Here's how the part is built. I have some questions about the finished solid (model axes, mm). Face numbers are marked on the shaded views. Give positions to 0.01 mm unless a question says otherwise; leave off trailing zeros. Write each loop counter-clockwise with the first axis right and the second up, starting at its lowest first coordinate (ties: lowest second). Pieces come first, ordered by that corner, then holes. Notation, with made-up numbers: (64, -32.75) - (81, -32.75) arc R11 cw to (81, -22.75) - close; hole circle Ø9 at (-9.75, -2). An arc over 180 degrees is marked (long way). Write each question's results on one line, items separated by ' | '. Start each with the question number.
Item 1: Suppose I cut it at B-B on z = -70. List the corners of the cut face in (x, y) for me.
Item 2: Will these pins go through, and if not, where does the flat tip stop? P1, Ø5, axis at x = -70, z = -70, coming from the -Y side; P2, Ø1.9, axis at x = -11, z = -11, coming from the +Y side; P3, Ø3, axis at y = 9, z = -67.5, coming from the -X side.
Item 3: Please list where these lines run through material, in increasing order: line 1 along X through (y, z) = (8.75, -70); line 2 along X through (y, z) = (9, -8).
Item 4: Suppose I cut it at A-A on y = 6.5. List the corners of the cut face in (x, z) for me, then the cut area to 3 significant figures.
Item 5: Suppose I cut it at C-C on x = -70. List the corners of the cut face in (y, z) for me, then the cut area to 3 significant figures.
Item 6: We'd pull the mould along X, two halves only. Please class the marked faces 1 and 2: +X half, -X half, draft (parallel to the pull), parting line (faces both ways), or undercut.
Item 7: Suppose I cut it at D-D on z = -16. List the corners of the cut face in (x, y) for me, then the cut area to 3 significant figures.
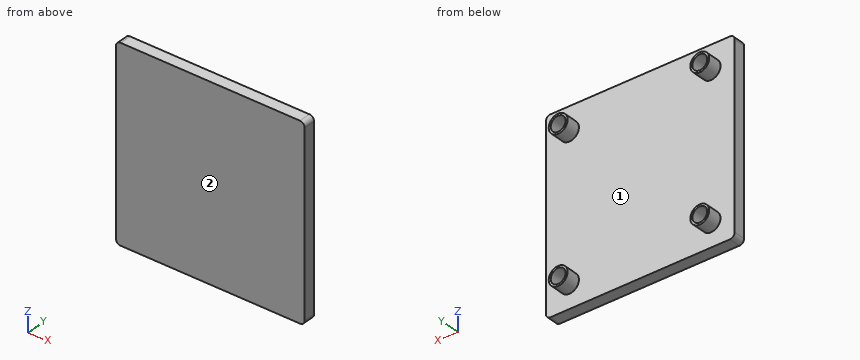
Autodesk Inventor part; units mm, degrees
ref_plane "YZ Plane" through (0, 0, 0) normal (1, 0, 0) x (0, 1, 0)
ref_plane "XZ Plane" through (0, 0, 0) normal (0, 1, 0) x (-1, 0, 0)
ref_plane "XY Plane" through (0, 0, 0) normal (0, 0, 1) x (1, 0, 0)
sketch "Sketch1" plane through (0, 0, 0) normal (0, 1, 0) x (-1, 0, 0)
  line L0 (0, 0) -> (80, 0)
  line L1 (80, 0) -> (80, -80)
  line L2 (80, -80) -> (0, -80)
  line L3 (0, -80) -> (0, 0)
  dimension "d0" = 80
extrude "Extrusion1" add sketch "Sketch1" along normal blind 5
fillet "Fillet1" radius 2 4 edges at (-80, 2.5, 0) (-80, 2.5, -80) (0, 2.5, -80) (0, 2.5, 0)
sketch "Sketch2" plane through (0, 5, 0) normal (0, 1, 0) x (1, 0, 0)
  line L0 (-10, 10) -> (-70, 10) construction
  line L1 (-70, 10) -> (-70, 70) construction
  line L2 (-70, 70) -> (-10, 70) construction
  line L3 (-10, 70) -> (-10, 10) construction
  line L4 (0, 2) -> (0, 78) construction
  line L5 (-78, 0) -> (-2, 0) construction
  circle A0 centre (-70, 10) radius 3.15
  circle A1 centre (-70, 70) radius 3.15
  circle A2 centre (-10, 70) radius 3.15
  circle A3 centre (-10, 10) radius 3.15
  circle A4 centre (-70, 10) radius 4
  circle A5 centre (-70, 70) radius 4
  circle A6 centre (-10, 70) radius 4
  circle A7 centre (-10, 10) radius 4
  point P0 (0, 0)
  dimension "d4" = 60
  dimension "d5" = 10
  dimension "d6" = 10
  dimension "d7" = 6.3
  dimension "d8" = 8
extrude "Extrusion2" add sketch "Sketch2" along normal blind 6
equation "\"d0\" = cradle_width"
equation "\"d4\" = rod_dist"
equation "\"d5\" = 0.5 * cradle_width - 0.5 * rod_dist"
equation "\"d6\" = 0.5 * cradle_width - 0.5 * rod_dist"
equation "\"d7\" = rod_diameter + rod_tolerance"
equation "\"d8\" = post_diameter"
equation "\"cradle_width\" = 80"
equation "\"rod_diameter\" = 6"
equation "\"rod_tolerance\" = 0.3"
equation "\"post_diameter\" = 8"
equation "\"rod_dist\" = 60"
properties part number "cradle_top"
Checked values:
1) outline: (-80, 0) - (0, 0) - (0, 5) - (-6, 5) - (-6, 11) - (-6.85, 11) - (-6.85, 5) - (-13.15, 5) - (-13.15, 11) - (-14, 11) - (-14, 5) - (-66, 5) - (-66, 11) - (-66.85, 11) - (-66.85, 5) - (-73.15, 5) - (-73.15, 11) - (-74, 11) - (-74, 5) - (-80, 5) - close
2) P1: stops at y = 0 | P2: stops at y = 5 | P3: stops at x = -73.87
3) line 1: x = -74 to -73.15, -66.85 to -66, -14 to -13.15, -6.85 to -6 | line 2: x = -73.46 to -72.43, -67.57 to -66.54, -13.46 to -12.43, -7.57 to -6.54
4) outline: circle Ø8 at (-70, -70); circle Ø8 at (-70, -10); circle Ø8 at (-10, -70); circle Ø8 at (-10, -10); hole circle Ø6.3 at (-70, -70); hole circle Ø6.3 at (-70, -10); hole circle Ø6.3 at (-10, -70); hole circle Ø6.3 at (-10, -10) | area: 76.4 mm^2
5) outline: (0, -80) - (5, -80) - (5, -74) - (11, -74) - (11, -73.15) - (5, -73.15) - (5, -66.85) - (11, -66.85) - (11, -66) - (5, -66) - (5, -14) - (11, -14) - (11, -13.15) - (5, -13.15) - (5, -6.85) - (11, -6.85) - (11, -6) - (5, -6) - (5, 0) - (0, 0) - close | area: 420 mm^2
6) face 1: undercut | face 2: draft
7) outline: (-80, 0) - (0, 0) - (0, 5) - (-80, 5) - close | area: 400 mm^2
